from build123d import *


with BuildPart() as part:
    # Sweep3: sweep along a path in Sketch3
    with BuildLine(Plane(origin=(0, 0, 0), x_dir=(0, 0, -1), z_dir=(1, 0, 0))) as sweep3_path:
        Line((0, 0), (-36.5379, 0))
    # Sketch2 → Sweep3 (sweep)
    with BuildSketch(Plane.XY):
        Polygon((0, 0), (6.35, 0), (6.35, -7.9375), (7.9375, -7.9375), (7.9375, 1.5875), (-1.5875, 1.5875), (-1.5875, -7.9375), (0, -7.9375), align=None)
    sweep(path=sweep3_path.line)


solid = part.part
Geometry check sheet. Reference: the model listing, model coordinates, mm. A direction names the side the tool comes from. Give positions to 0.01 mm unless a question says otherwise; leave off trailing zeros. Loops run counter-clockwise (first coordinate to the right, second up) from the corner with the lowest first, then second, coordinate; pieces in that order, holes last. Notation, with made-up numbers: (66.25, -16) -> (75.25, -16) arc R21 cw to (75.25, 7) -> close; hole circle Ø9 at (40.25, 49). An arc over 180 degrees is marked (long way). Answer in a Markdown table with one row per item. Add a question column.
1) Material ranges on probe 1 along X at (y, z) = (-4.75, 3); probe 2 along Y at (x, z) = (4.5, 28.5), recorded low to high. Write a range as from..to.
2) Draft check along X on faces 3 (the face through (7.938, -3, 19)), 4 (the face through (-1, -7.938, 19)), 5 (the face through (3, 0, 19)), 6 (the face through (6.35, -4, 19)). Enter one of: pulls with the +X half, pulls with the -X half, needs draft (parallel to the pull), parting line crosses it, or undercut.
3) Cross-section at B-B on z = 8. Record the boundary of the cut face in (x, y).
4) Set-up check for faces 1 (the face through (0, -4, 19)), 2 (the face through (3, 1.588, 19)): record each of +Z, -Z, +X, -X, +Y, -Y from which the full face is reachable in a straight line by a thin tool's end or side.
5) Cross-section at C-C on x = 5.25. Record the boundary of the cut face in (y, z), and give its area (3 significant figures).
6) Cross-section at A-A on y = -4. Record the boundary of the cut face in (x, z), and give its area (3 significant figures).
Outcome:
| question | item | result |
|---|---|---|
| 1 | probe 1 | x = -1.59..0, 6.35..7.94 |
| 1 | probe 2 | y = 0..1.59 |
| 2 | face 3 | pulls with the +X half |
| 2 | face 4 | needs draft |
| 2 | face 5 | undercut |
| 2 | face 6 | undercut |
| 3 | outline | (-1.59, -7.94) -> (0, -7.94) -> (0, 0) -> (6.35, 0) -> (6.35, -7.94) -> (7.94, -7.94) -> (7.94, 1.59) -> (-1.59, 1.59) -> close |
| 4 | face 1 | +Z, -Z, -Y |
| 4 | face 2 | +Z, -Z, +X, -X, +Y |
| 5 | outline | (0, 0) -> (1.59, 0) -> (1.59, 36.54) -> (0, 36.54) -> close |
| 5 | area | 58.0 mm^2 |
| 6 | outline | (-1.59, 0) -> (0, 0) -> (0, 36.54) -> (-1.59, 36.54) -> close; (6.35, 0) -> (7.94, 0) -> (7.94, 36.54) -> (6.35, 36.54) -> close |
| 6 | area | 116 mm^2 |
